Could you check a few things on this model? Use its own coordinates, in mm. A direction names the side the tool comes from. Coordinates: 2 decimals unless noted, no trailing zeros. Write each loop counter-clockwise with the first axis right and the second up, starting at its lowest first coordinate (ties: lowest second). Pieces come first, ordered by that corner, then holes.
Item 1: Thinking about a two-plate mould opening in Z: for faces 1 (the flat face through (-14, 50.8, -192)), 2 (the flat face through (14, 75, -104.14)), 3 (the flat face through (-965.2, 28, 8)), 4 (the flat face through (-14, 25, 571.5)), which applies, +Z half, -Z half, draft (parallel to the pull), parting line (faces both ways), or undercut?
Item 2: I want a section at B-B on y = 69. Please give me the cut outline in (x, z).
Item 3: For P1, Ø4, axis at x = -311, z = 246.5, coming from the +Y side; P2, Ø3, axis at x = 155.5, y = 86, coming from the -Z side; P3, Ø10, axis at x = -101.6, z = -130.175, coming from the -Y side, each with a flat end and sliding along its axis, tell me the tip position at first contact or that it passes through.
Item 4: I want a section at C-C on z = -319. Please give me the cut outline in (x, y), then the cut area to 3 significant figures.
Item 5: I want a section at A-A on x = -35.5. Please give me the cut outline in (y, z), then the cut area to 3 significant figures.
Item 6: If I drill on probe 1 along Z at (x, y) = (-101, 100); probe 2 along Y at (x, z) = (-538, -134); probe 3 along Z at (x, y) = (-343.5, 70), over which ranges is the centre line in solid material (lowest first)?
Item 7: Which directions (+Z, -Z, +X, -X, +Y, -Y) give clear straight access to the entire face, cutting with the end or side of a thin tool? Please do faces 5 (the flat face through (14, 75, -276.86)), 6 (the flat face through (-13, 3.048, -7)), 7 (the flat face through (14, 101.6, -192)), 8 (the flat face through (-14, 50.8, -427)), 9 (the flat face through (14, 77, -101.6)).
from build123d import *

# Parameters (mm, degrees)
SKETCH1_W           = 1930.4
SKETCH1_H           = 1143
BOSS_EXTRUDE1_DEPTH = 50.8
SKETCH2_W           = 1861.76231229
SKETCH2_H           = 1069.640341316
CUT_EXTRUDE1_DEPTH  = 3.048
BOSS_EXTRUDE3_DEPTH = 1930.4
CUT_EXTRUDE2_REACH  = 1128.297
SKETCH4_R           = 3.175


with BuildPart() as part:
    # Sketch1 → Boss-Extrude1 (new body)
    with BuildSketch(Plane(origin=(0, 0, 0), x_dir=(1, 0, 0), z_dir=(0, 1, 0))):
        Rectangle(SKETCH1_W, SKETCH1_H)
    extrude(amount=BOSS_EXTRUDE1_DEPTH)

    # Sketch2 → Cut-Extrude1 (cut)
    with BuildSketch(Plane(origin=(0, 0, 0), x_dir=(1, 0, 0), z_dir=(0, 1, 0))):
        Rectangle(SKETCH2_W, SKETCH2_H)
    extrude(amount=CUT_EXTRUDE1_DEPTH, mode=Mode.SUBTRACT)

    # Sketch3 → Boss-Extrude3 (add, through all)
    with BuildSketch(Plane(origin=(965.2, 0, 0), x_dir=(0, 0, -1), z_dir=(1, 0, 0))):
        Polygon((101.6, 50.8), (104.14, 50.8), (104.14, 99.06), (276.86, 99.06), (276.86, 50.8), (279.4, 50.8), (279.4, 101.6), (101.6, 101.6), align=None)
    extrude(amount=-BOSS_EXTRUDE3_DEPTH)

    # Sketch4 → Cut-Extrude2 (cut, up to next)
    with BuildSketch(Plane(origin=(0, 101.6, 0), x_dir=(1, 0, 0), z_dir=(0, 1, 0)), mode=Mode.PRIVATE) as cut_extrude2_sk1:
        with Locations(Location((101.6, 130.175, 0), (0, 0, 270))):
            Circle(SKETCH4_R)
    cut_extrude2_tool1 = extrude(cut_extrude2_sk1.sketch, amount=-CUT_EXTRUDE2_REACH, mode=Mode.PRIVATE) & part.part
    # Sketch4 → Cut-Extrude2 (cut, up to next)
    with BuildSketch(Plane(origin=(0, 101.6, 0), x_dir=(1, 0, 0), z_dir=(0, 1, 0)), mode=Mode.PRIVATE) as cut_extrude2_sk2:
        with Locations(Location((-101.6, 130.175, 0), (0, 0, 270))):
            Circle(SKETCH4_R)
    cut_extrude2_tool2 = extrude(cut_extrude2_sk2.sketch, amount=-CUT_EXTRUDE2_REACH, mode=Mode.PRIVATE) & part.part
    # Sketch4 → Cut-Extrude2 (cut, up to next)
    with BuildSketch(Plane(origin=(0, 101.6, 0), x_dir=(1, 0, 0), z_dir=(0, 1, 0)), mode=Mode.PRIVATE) as cut_extrude2_sk3:
        with Locations(Location((-101.6, 257.175, 0), (0, 0, 270))):
            Circle(SKETCH4_R)
    cut_extrude2_tool3 = extrude(cut_extrude2_sk3.sketch, amount=-CUT_EXTRUDE2_REACH, mode=Mode.PRIVATE) & part.part
    # Sketch4 → Cut-Extrude2 (cut, up to next)
    with BuildSketch(Plane(origin=(0, 101.6, 0), x_dir=(1, 0, 0), z_dir=(0, 1, 0)), mode=Mode.PRIVATE) as cut_extrude2_sk4:
        with Locations(Location((101.6, 257.175, 0), (0, 0, 270))):
            Circle(SKETCH4_R)
    cut_extrude2_tool4 = extrude(cut_extrude2_sk4.sketch, amount=-CUT_EXTRUDE2_REACH, mode=Mode.PRIVATE) & part.part
    add(cut_extrude2_tool1.solids().sort_by_distance((101.6, 101.6, -130.175))[0], mode=Mode.SUBTRACT)
    add(cut_extrude2_tool2.solids().sort_by_distance((-101.6, 101.6, -130.175))[0], mode=Mode.SUBTRACT)
    add(cut_extrude2_tool3.solids().sort_by_distance((-101.6, 101.6, -257.175))[0], mode=Mode.SUBTRACT)
    add(cut_extrude2_tool4.solids().sort_by_distance((101.6, 101.6, -257.175))[0], mode=Mode.SUBTRACT)


solid = part.part
Response values:
1. face 1: undercut
1. face 2: undercut
1. face 3: draft
1. face 4: +Z half
2. outline: (-965.2, -279.4) - (965.2, -279.4) - (965.2, -276.86) - (-965.2, -276.86) - close; (-965.2, -104.14) - (965.2, -104.14) - (965.2, -101.6) - (-965.2, -101.6) - close
3. P1: stops at y = 50.8
3. P2: stops at z = -279.4
3. P3: stops at y = 3.05
4. outline: (-965.2, 0) - (-930.88, 0) - (-930.88, 3.05) - (930.88, 3.05) - (930.88, 0) - (965.2, 0) - (965.2, 50.8) - (-965.2, 50.8) - close
4. area: 92,400 mm2
5. outline: (0, -571.5) - (50.8, -571.5) - (50.8, -279.4) - (101.6, -279.4) - (101.6, -101.6) - (50.8, -101.6) - (50.8, 571.5) - (0, 571.5) - (0, 534.82) - (3.05, 534.82) - (3.05, -534.82) - (0, -534.82) - close; hole (50.8, -276.86) - (99.06, -276.86) - (99.06, -104.14) - (50.8, -104.14) - close
5. area: 55,500 mm2
6. probe 1: z = -279.4 to -260.29, -254.06 to -133.29, -127.06 to -101.6
6. probe 2: y = 3.05 to 50.8, 99.06 to 101.6
6. probe 3: z = -279.4 to -276.86, -104.14 to -101.6
7. face 5: +X, -X
7. face 6: -Y
7. face 7: +Z, -Z, +X, -X, +Y
7. face 8: -Z, +X, -X, +Y
7. face 9: +Z, +X, -X, +Y
